Can you work these out from the model? Positions are in its coordinate system, mm. Face numbers are marked on the shaded views. A direction names the side the tool comes from. Give positions to 0.01 mm unless a question says otherwise; leave off trailing zeros. Loops run counter-clockwise (first coordinate to the right, second up) from the corner with the lowest first, then second, coordinate; pieces in that order, holes last. Notation, with made-up numbers: (21, 2) - (42, 2) arc R9 cw to (42, 15) - close; hole circle Ø3 at (79.25, 50.5). An arc over 180 degrees is marked (long way). Answer as a JSON object with one key per item and string values.
```python
from build123d import *

# Parameters (mm, degrees)
SKETCH2_R           = 50
BOSS_EXTRUDE1_DEPTH = 3
CUT_EXTRUDE1_DEPTH  = 38.1
SKETCH9_W           = 8
SKETCH9_H           = 8
BOSS_EXTRUDE2_DEPTH = 38.1
SKETCH10_R          = 3
CUT_EXTRUDE2_DEPTH  = 3


with BuildPart() as part:
    # Sketch2 → Boss-Extrude1 (new body)
    with BuildSketch(Plane(origin=(0, 0, 0), x_dir=(1, 0, 0), z_dir=(0, 1, 0))):
        with Locations(Location((0, 0, 0), (0, 0, 270))):
            Circle(SKETCH2_R)
    extrude(amount=BOSS_EXTRUDE1_DEPTH)

    # Sketch6 → Cut-Extrude1 (cut)
    with BuildSketch(Plane(origin=(0, 3, 0), x_dir=(1, 0, 0), z_dir=(0, 1, 0))):
        Polygon((-43.65, 24.386010334), (-43.65, -24.386010334), (-50, -24.386010334), (-50, 0), (-50, 24.386010334), align=None)
        Polygon((43.65, 24.386010334), (43.65, -24.386010334), (50, -24.386010334), (50, 0), (50, 24.386010334), align=None)
    extrude(amount=-CUT_EXTRUDE1_DEPTH, mode=Mode.SUBTRACT)

    # Sketch9 → Boss-Extrude2 (add)
    with BuildSketch(Plane(origin=(0, 3, 0), x_dir=(1, 0, 0), z_dir=(0, 1, 0))):
        with Locations((-39.65, 20.386010334)):
            Rectangle(SKETCH9_W, SKETCH9_H)
        with Locations((39.65, 20.386010334)):
            Rectangle(SKETCH9_W, SKETCH9_H)
        with Locations((39.65, -20.386010334)):
            Rectangle(SKETCH9_W, SKETCH9_H)
        with Locations((-39.65, -20.386010334)):
            Rectangle(SKETCH9_W, SKETCH9_H)
    extrude(amount=BOSS_EXTRUDE2_DEPTH)

    # Sketch10 → Cut-Extrude2 (cut)
    with BuildSketch(Plane(origin=(0, 0, 0), x_dir=(-1, 0, 0), z_dir=(0, -1, 0))):
        with Locations(Location((31.35, -24.386010334, 0), (0, 0, 90))):
            Circle(SKETCH10_R)
        with Locations(Location((31.35, 24.386010334, 0), (0, 0, 90))):
            Circle(SKETCH10_R)
        with Locations(Location((-31.35, 24.386010334, 0), (0, 0, 90))):
            Circle(SKETCH10_R)
        with Locations(Location((-31.35, -24.386010334, 0), (0, 0, 90))):
            Circle(SKETCH10_R)
    extrude(amount=-CUT_EXTRUDE2_DEPTH, mode=Mode.SUBTRACT)


solid = part.part
```
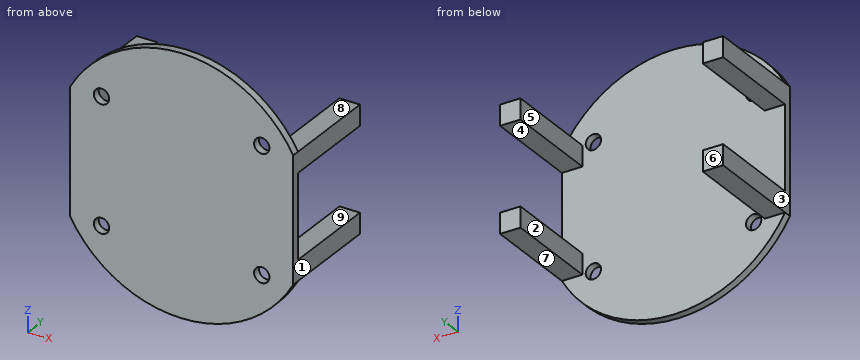
1) If we mould it in two halves opening along X, with no side actions, what happens to the marked faces 1, 2, 3 and 4? For each: released by +X, released by -X, zero draft, split by the parting line, or undercut.
Check sheet entries:
{"face 1": "released by +X", "face 2": "undercut", "face 3": "released by -X", "face 4": "zero draft"}
2) I'm going to push flat-ended pins straight in: P1, Ø4, axis at y = 25, z = -28, coming from the -X side; P2, Ø6.5, axis at x = 40.5, y = 25, coming from the -Z side; P3, Ø10, axis at x = -2, z = 19, coming from the +Y side; P4, Ø4, axis at x = 40, y = 30, coming from the +Z side. Where does each tip first touch, or does it pass through?
Check sheet entries:
{"P1": "through", "P2": "z = -24.39", "P3": "y = 3", "P4": "z = 24.39"}
3) Imagine slicing it at D-D on x = -4.5. Write out the boundary of the cut face in (y, z).
Check sheet entries:
{"outline": "(0, -49.8) - (3, -49.8) - (3, 49.8) - (0, 49.8) - close"}
4) I need wall thicknesses on L1, parallel to Z at x = -39, y = 6.5; L2, parallel to X at y = 22, z = -24; L3, parallel to Y at x = 6.5, z = 12.5. Which ranges of each line are inside material? Lowest first, please.
Check sheet entries:
{"L1": "-24.39 to -16.39, 16.39 to 24.39", "L2": "-43.65 to -35.65, 35.65 to 43.65", "L3": "0 to 3"}
5) Imagine slicing it at B-B on y = 9.5. Write out the boundary of the cut face in (x, z), and give its area (3 significant figures).
Check sheet entries:
{"outline": "(-43.65, -24.39) - (-35.65, -24.39) - (-35.65, -16.39) - (-43.65, -16.39) - close; (-43.65, 16.39) - (-35.65, 16.39) - (-35.65, 24.39) - (-43.65, 24.39) - close; (35.65, -24.39) - (43.65, -24.39) - (43.65, -16.39) - (35.65, -16.39) - close; (35.65, 16.39) - (43.65, 16.39) - (43.65, 24.39) - (35.65, 24.39) - close", "area": "256 mm2"}
6) Imagine slicing it at C-C on x = 14. Write out the boundary of the cut face in (y, z), and give its area (3 significant figures).
Check sheet entries:
{"outline": "(0, -48) - (3, -48) - (3, 48) - (0, 48) - close", "area": "288 mm2"}
7) Which directions (+Z, -Z, +X, -X, +Y, -Y) give clear straight access to the entire face, cutting with the end or side of a thin tool? Please do the marked faces 5, 6, 7, 8 and 9.
Check sheet entries:
{"face 5": "+Z, -Z, +Y", "face 6": "+Z, -Z, +X, -X, +Y", "face 7": "-Z, +X, -X, +Y", "face 8": "+Z, +X, -X, +Y", "face 9": "+X, -X, +Y"}
8) Imagine slicing it at A-A on x = 31.35. Write out the boundary of the cut face in (y, z), and give its area (3 significant figures).
Check sheet entries:
{"outline": "(0, -38.95) - (3, -38.95) - (3, -27.39) - (0, -27.39) - close; (0, -21.39) - (3, -21.39) - (3, 21.39) - (0, 21.39) - close; (0, 27.39) - (3, 27.39) - (3, 38.95) - (0, 38.95) - close", "area": "198 mm2"}
